Answer from the drawing. Dimensions are ordinates in mm from the lowest x, y and z of the part. Coordinates: 2 decimals unless noted, no trailing zeros. Write each loop counter-clockwise with the first axis right and the second up, starting at its lowest first coordinate (ties: lowest second). Pieces come first, ordered by that corner, then holes. Notation, with made-up numbers: (14.5, 70.5) -> (70.5, 70.5) arc R15 ccw to (70.5, 76.5) -> close; hole circle Ø2 at (77.25, 57). An arc over 180 degrees is marked (long way). Answer as a JSON object with one key per item and string values. Group by question number.
(1) Find section D-D (y = 82). Give the vertices of the cut face in (x, z).
(2) Find section C-C (z = 6). Give the vertices of the cut face in (x, y), then the cut area to 3 significant figures.
(3) Find section B-B (x = 113). Give the vertices of the cut face in (y, z).
(4) Find section A-A (y = 35). Give the vertices of the cut face in (x, z).
(5) A flat-ended cylindrical pin translates along its axis: P1, Ø18, axis at x = 113, y = 76, coming from the -Z side. Find the tip coordinate at first contact, or state that the pin passes through.
(6) For a pull along Y with two mould halves and no side action, classify the marked faces 1, 2 and 3 as +Y half, -Y half, draft (parallel to the pull), parting line (faces both ways), or undercut.
(7) Straight lines are drawn through the part: L1, parallel to Y at x = 113, z = 36.5; L2, parallel to X at y = 35, z = 50.5; L3, parallel to X at y = 44, z = 48. For each, find the intervals that lie inside material, in ascending order.
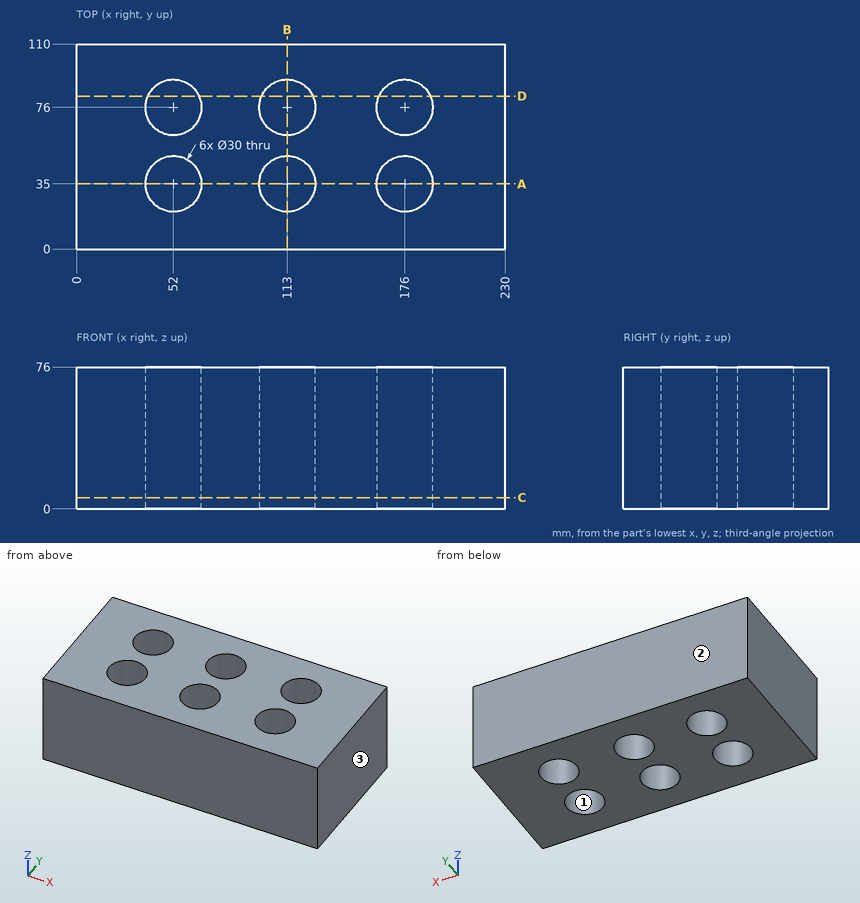
Results below:
{
 "1": {"outline": "(0, 0) -> (38.25, 0) -> (38.25, 76) -> (0, 76) -> close; (65.75, 0) -> (99.25, 0) -> (99.25, 76) -> (65.75, 76) -> close; (126.75, 0) -> (162.25, 0) -> (162.25, 76) -> (126.75, 76) -> close; (189.75, 0) -> (230, 0) -> (230, 76) -> (189.75, 76) -> close"},
 "2": {"outline": "(0, 0) -> (230, 0) -> (230, 110) -> (0, 110) -> close; hole circle Ø30 at (52, 35); hole circle Ø30 at (52, 76); hole circle Ø30 at (113, 35); hole circle Ø30 at (113, 76); hole circle Ø30 at (176, 35); hole circle Ø30 at (176, 76)", "area": "21,100 mm2"},
 "3": {"outline": "(0, 0) -> (20, 0) -> (20, 76) -> (0, 76) -> close; (50, 0) -> (61, 0) -> (61, 76) -> (50, 76) -> close; (91, 0) -> (110, 0) -> (110, 76) -> (91, 76) -> close"},
 "4": {"outline": "(0, 0) -> (37, 0) -> (37, 76) -> (0, 76) -> close; (67, 0) -> (98, 0) -> (98, 76) -> (67, 76) -> close; (128, 0) -> (161, 0) -> (161, 76) -> (128, 76) -> close; (191, 0) -> (230, 0) -> (230, 76) -> (191, 76) -> close"},
 "5": {"P1": "passes through"},
 "6": {"face 1": "undercut", "face 2": "+Y half", "face 3": "draft"},
 "7": {"L1": "y = 0 to 20, 50 to 61, 91 to 110", "L2": "x = 0 to 37, 67 to 98, 128 to 161, 191 to 230", "L3": "x = 0 to 40, 64 to 101, 125 to 164, 188 to 230"}
}
